CAD build for the part. Positions are in the model's coordinates, mm. Round coordinates to 2 decimals unless told otherwise and drop trailing zeros. Loops run counter-clockwise (first coordinate to the right, second up) from the corner with the lowest first, then second, coordinate; pieces in that order, holes last.
```python
from build123d import *

# Parameters (mm, degrees)
EXTRUDE_1_DEPTH = 0.5


with BuildPart() as part:
    # Эскиз1 → Вытянуть1 (new body)
    with BuildSketch(Plane.XY):
        with BuildLine():
            Line((2.063762187, -60), (10.569656745, -60))
            ThreePointArc((10.569656745, -60), (51.430925196, -12.664111557), (92.292193648, -60))
            Line((92.292193648, -60), (98.287869977, -60))
            Line((98.287869977, -60), (98.287869977, 0))
            Line((98.287869977, 0), (2.063762187, 0))
            Line((2.063762187, 0), (2.063762187, -60))
        make_face()
    extrude(amount=EXTRUDE_1_DEPTH)


solid = part.part
```
Item 1: Cut at D-D, the plane x = 41.5. Give the cut face in (y, z).
Answers follow:
outline: (-13.88, 0) - (0, 0) - (0, 0.5) - (-13.88, 0.5) - close
Item 2: Two-plate mould, pull along X, no slides. Class faces 1 (the flat face through (50, -10, 0)), 2 (the cylindrical face through (50.438, -12.676, 0.246)): released by +X, released by -X, zero draft, split by the parting line, or undercut.
Answers follow:
face 1: zero draft
face 2: undercut
Item 3: Cut at B-B, the plane z = 0.2. Give the cut face in (x, y), plus the area to 3 significant figures.
Answers follow:
outline: (2.06, -60) - (10.57, -60) arc R41.3 cw (long way) to (92.29, -60) - (98.29, -60) - (98.29, 0) - (2.06, 0) - close
area: 2,600 mm2
Item 4: Cut at C-C, the plane y = -42. Give the cut face in (x, z).
Answers follow:
outline: (2.06, 0) - (11.9, 0) - (11.9, 0.5) - (2.06, 0.5) - close; (90.96, 0) - (98.29, 0) - (98.29, 0.5) - (90.96, 0.5) - close
Item 5: Probe line 1 (X direction, y = -55, z = 0.45); line 2 (X direction, y = -50.5, z = 0.15); line 3 (Y direction, x = 64, z = 0.35). List the from-to ranges inside material, lowest first.
Answers follow:
line 1: x = 2.06 to 10.14, 92.72 to 98.29
line 2: x = 2.06 to 10.27, 92.59 to 98.29
line 3: y = -14.62 to 0
Item 6: Cut at A-A, the plane y = -30. Give the cut face in (x, z), plus the area to 3 significant figures.
Answers follow:
outline: (2.06, 0) - (17.79, 0) - (17.79, 0.5) - (2.06, 0.5) - close; (85.07, 0) - (98.29, 0) - (98.29, 0.5) - (85.07, 0.5) - close
area: 14.5 mm2
